from build123d import *

# Parameters (mm, degrees)
SKETCH_1_W                = 44.5
SKETCH_1_H                = 182
EXTRUDE_1_DEPTH           = 20
FILLET_1_R                = 8
HOLE_WIZARD_1_4_201_D     = 5.1054
HOLE_WIZARD_1_4_201_DEPTH = 10
EXTRUDE_2_DEPTH           = 20
FILLET_2_R                = 100
CUT_EXTRUDE_1_REACH       = 180.298
CUT_EXTRUDE_2_REACH       = 180.781
SKETCH_7_R                = 5.25
EXTRUDE_3_DEPTH           = 20
FILLET_7_R                = 4
SKETCH_10_W               = 2
SKETCH_10_H               = 17.136672327
EXTRUDE_4_DEPTH           = 20
CUT_EXTRUDE_3_REACH       = 182.814
SKETCH_11_R               = 4.1
CUT_EXTRUDE_START         = -20
SKETCH_12_W               = 51.6
SKETCH_12_H               = 2.481518881
CUT_EXTRUDE_4_DEPTH       = 20
EXTRUDE_5_DEPTH           = 20


with BuildPart() as part:
    # Эскиз1 → Бобышка-Вытянуть1 (new body)
    with BuildSketch(Plane.XY):
        with Locations((20.25, 81)):
            Rectangle(SKETCH_1_W, SKETCH_1_H)
        with BuildLine():
            Line((8, 0), (32.5, 0))
            ThreePointArc((32.5, 0), (36.5, -4), (40.5, 0))
            Line((40.5, 0), (40.5, 170))
            Line((40.5, 170), (0, 170))
            Line((0, 170), (0, 0))
            ThreePointArc((0, 0), (4, -4), (8, 0))
        make_face(mode=Mode.SUBTRACT)
    extrude(amount=EXTRUDE_1_DEPTH)

    # Скругление1
    fillet_1_edges = [part.edges().sort_by_distance(p)[0] for p in [
        (8, 0, 10),
        (32.5, 0, 10),
        (42.5, -10, 10),
        (-2, -10, 10),
    ]]
    fillet(fillet_1_edges, radius=FILLET_1_R)

    # Отверстие обработанное метчиком 1/4-201
    with Locations(Plane(origin=(0, -10, 0), x_dir=(-1, 0, 0), z_dir=(0, -1, 0))):
        with Locations((-20.25, -10)):
            Hole(HOLE_WIZARD_1_4_201_D / 2, depth=HOLE_WIZARD_1_4_201_DEPTH)

    # Эскиз5 → Бобышка-Вытянуть2 (add)
    with BuildSketch(Plane.XY.offset(20)):
        with BuildLine():
            Line((-7.1, 155), (-7.1, 136))
            ThreePointArc((-7.1, 136), (-5.807601094, 124.936546651), (-2, 114.468859761))
            Line((-2, 114.468859761), (-2, 110.317515696))
            ThreePointArc((-2, 110.317515696), (-7.29232304, 122.677087406), (-9.1, 136))
            Line((-9.1, 136), (-9.1, 155))
            Line((-9.1, 155), (-7.1, 155))
        make_face()
    extrude(amount=-EXTRUDE_2_DEPTH)

    # Скругление2
    fillet_2_edges = [part.edges().sort_by_distance(p)[0] for p in [
        (-2, 110.317515696, 10),
    ]]
    fillet(fillet_2_edges, radius=FILLET_2_R)

    # Эскиз6 → Вырез-Вытянуть1 (cut, up to next)
    with BuildSketch(Plane.XY.offset(20), mode=Mode.PRIVATE) as cut_extrude_1_sk1:
        Polygon((0, 170), (0, 114.468859761), (-2, 114.468859761), (-2, 170), (-2, 172), (42.5, 172), (42.5, 170), align=None)
    cut_extrude_1_tool1 = extrude(cut_extrude_1_sk1.sketch, amount=-CUT_EXTRUDE_1_REACH, mode=Mode.PRIVATE) & part.part
    add(cut_extrude_1_tool1.solids().sort_by_distance((-0.72733, 142.23443, 20))[0], mode=Mode.SUBTRACT)

    # Эскиз7 → Вырез-Вытянуть2 (cut, up to next)
    with BuildSketch(Plane.ZY.offset(9.1), mode=Mode.PRIVATE) as cut_extrude_2_sk1:
        with Locations((10, 145.426275666)):
            Circle(SKETCH_7_R)
    cut_extrude_2_tool1 = extrude(cut_extrude_2_sk1.sketch, amount=-CUT_EXTRUDE_2_REACH, mode=Mode.PRIVATE) & part.part
    add(cut_extrude_2_tool1.solids().sort_by_distance((-9.1, 145.426276, 10))[0], mode=Mode.SUBTRACT)

    # Эскиз9 → Бобышка-Вытянуть3 (add)
    with BuildSketch(Plane.XY.offset(20)):
        with BuildLine():
            Line((-7.051971502, 133.853274797), (0, 133.853274797))
            Line((0, 133.853274797), (0, 114.468859761))
            Line((0, 114.468859761), (-2, 114.468859761))
            ThreePointArc((-2, 114.468859761), (-5.548456035, 123.894590796), (-7.051971502, 133.853274797))
        make_face()
    extrude(amount=-EXTRUDE_3_DEPTH)

    # Скругление7
    fillet_7_edges = [part.edges().sort_by_distance(p)[0] for p in [
        (-7.051971502, 133.853274797, 10),
    ]]
    fillet(fillet_7_edges, radius=FILLET_7_R)

    # Эскиз10 → Бобышка-Вытянуть4 (add)
    with BuildSketch(Plane.XY.offset(20)):
        with Locations((-8.1, 163.568336164)):
            Rectangle(SKETCH_10_W, SKETCH_10_H)
    extrude(amount=-EXTRUDE_4_DEPTH)

    # Эскиз11 → Вырез-Вытянуть3 (cut, up to next)
    with BuildSketch(Plane.ZY.offset(9.1), mode=Mode.PRIVATE) as cut_extrude_3_sk1:
        with Locations((10, 162.426275666)):
            Circle(SKETCH_11_R)
    cut_extrude_3_tool1 = extrude(cut_extrude_3_sk1.sketch, amount=-CUT_EXTRUDE_3_REACH, mode=Mode.PRIVATE) & part.part
    add(cut_extrude_3_tool1.solids().sort_by_distance((-9.1, 162.426276, 10))[0], mode=Mode.SUBTRACT)

    # Эскиз12 → Вырез-Вытянуть4 (cut)
    with BuildSketch(Plane.XY.offset(20).offset(CUT_EXTRUDE_START)):
        with Locations((16.7, 170.895912887)):
            Rectangle(SKETCH_12_W, SKETCH_12_H)
    extrude(amount=CUT_EXTRUDE_4_DEPTH, mode=Mode.SUBTRACT)

    # Эскиз13 → Бобышка-Вытянуть5 (add)
    with BuildSketch(Plane.XY.offset(20)):
        with BuildLine():
            Line((36.5, 175.655153446), (-3.1, 175.655153446))
            ThreePointArc((-3.1, 175.655153446), (-7.342640687, 173.897794133), (-9.1, 169.655153446))
            Line((-9.1, 169.655153446), (-7.1, 169.655153446))
            ThreePointArc((-7.1, 169.655153446), (-5.928427125, 172.483580571), (-3.1, 173.655153446))
            Line((-3.1, 173.655153446), (36.5, 173.655153446))
            ThreePointArc((36.5, 173.655153446), (39.328427125, 172.483580571), (40.5, 169.655153446))
            Line((40.5, 169.655153446), (42.5, 169.655153446))
            ThreePointArc((42.5, 169.655153446), (40.742640687, 173.897794133), (36.5, 175.655153446))
        make_face()
    extrude(amount=-EXTRUDE_5_DEPTH)


solid = part.part
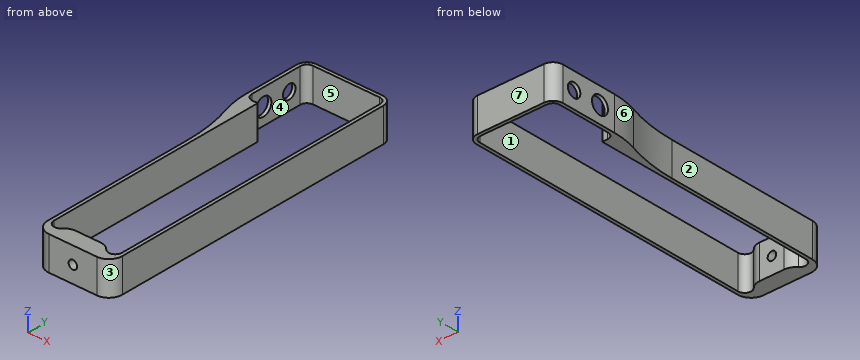
Design review of the part built by this model. Coordinates are the model's own, in mm. Face numbers are marked on the shaded views. A direction names the side the tool comes from. Give positions to 0.01 mm unless a question says otherwise; leave off trailing zeros. Write each loop counter-clockwise with the first axis right and the second up, starting at its lowest first coordinate (ties: lowest second). Pieces come first, ordered by that corner, then holes. Notation, with made-up numbers: M -31,87.25 L -8,87.25 A12 cw -8,104.25 Z; hole C 14.5,-13.75 d7. An arc over 180 degrees is marked long. Return JSON: item names as keys, results as strings. Group by question number.
Item 1: Clearance check with flat-ended pins moving along their axes: pin 1 Ø5 at (y, z) = (122.5, 5) entering from -X (3 decimals); pin 2 Ø8 at (x, z) = (-2.5, 10.5) entering from -Y; pin 3 Ø8 at (x, z) = (20.25, 10) entering from -Y; pin 4 Ø6 at (y, z) = (129.5, 10.5) entering from -X. State where each tip first meets the part, or that it passes through.
Item 2: Take a section at D-D (x = 31.5). Give the boundary of the cut face in (y, z).
Item 3: Take a section at A-A (y = 48). Give the boundary of the cut face in (x, z), plus the area to 3 significant figures.
Item 4: Take a section at C-C (z = 10). Count the separate pieces of the cut face and the enclosed holes in it, plus the area to 3 significant figures.
Item 5: Wall thickness on line 1 along X through (y, z) = (76.5, 14.5); line 2 along Y through (x, z) = (18.5, 12.75); line 3 along X through (y, z) = (-3.5, 10): over which ranges is each line inside the solid? List them lowest first.
Item 6: The part is to be moulded in two halves that separate along X. For the marked faces 4, 5, 6 and 7, say which applies: pulls with the +X half, pulls with the -X half, needs draft (parallel to the pull), parting line crosses it, or undercut.
Item 7: Take a section at B-B (x = 20.25). Give the boundary of the cut face in (y, z).
Item 8: Tool access review of the marked faces 1, 2 and 3: name each direction out of +Z, -Z, +X, -X, +Y, -Y from which nothing blocks a thin tool from reaching the whole face with its end or side.
Return value:
{
 "1": {"pin 1": "stops at x = -7.875", "pin 2": "stops at y = -8.61", "pin 3": "stops at y = -10", "pin 4": "stops at x = -8.98"},
 "2": {"outline": "M -10,0 L -1.04,0 L -1.04,20 L -10,20 Z; M 173.66,0 L 175.66,0 L 175.66,20 L 173.66,20 Z"},
 "3": {"outline": "M -2,0 L 0,0 L 0,20 L -2,20 Z; M 40.5,0 L 42.5,0 L 42.5,20 L 40.5,20 Z", "area": "80.0 mm2"},
 "4": {"separate pieces": "3", "enclosed holes": "0", "area": "1,190 mm2"},
 "5": {"line 1": "x = -2 to 0, 40.5 to 42.5", "line 2": "y = -10 to 0, 173.66 to 175.66", "line 3": "x = -1.86 to 2.06, 5.94 to 17.7, 22.8 to 34.56, 38.44 to 42.36"},
 "6": {"face 4": "undercut", "face 5": "undercut", "face 6": "pulls with the -X half", "face 7": "needs draft"},
 "7": {"outline": "M -10,0 L 0,0 L 0,7.45 L -10,7.45 Z; M -10,12.55 L 0,12.55 L 0,20 L -10,20 Z; M 173.66,0 L 175.66,0 L 175.66,20 L 173.66,20 Z"},
 "8": {"face 1": "+Z, -Z", "face 2": "+Z, -Z, -X, -Y", "face 3": "+Z, -Z, +X, -Y"}
}
